Input: part model. Units: mm. Frame: model coordinates. Face numbers are marked on the shaded views. A direction names the side the tool comes from. Coordinates: 2 decimals unless noted, no trailing zeros. Order: outer loops, then holes, each group sorted by start corner. A loop starts at its lowest first (then second) coordinate and runs counter-clockwise, first axis right, second up. Notation, with made-up numbers: (19, 50) -> (64, 50) arc R22 ccw to (64, 77) -> close; hole circle Ø2 at (-28.5, 37.5). An arc over 180 degrees is marked (long way). Answer as CSV lines item,"result".
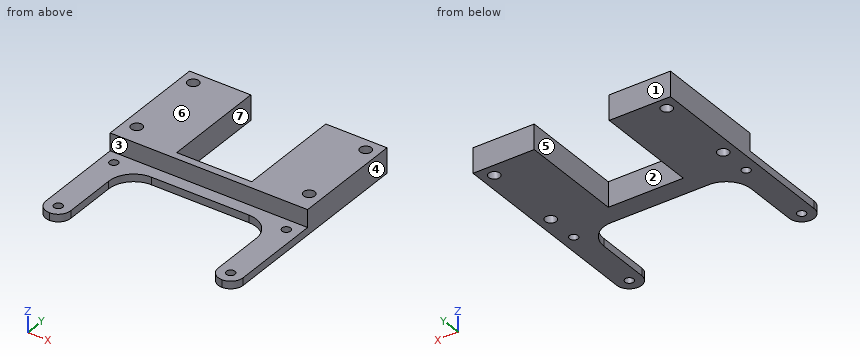
from build123d import *

# Parameters (mm, degrees)
BOSS_EXTRUDE1_DEPTH  = 3
FILLET1_R            = 10
FILLET2_R            = 5
M3_CLEARANCE_HOLE1_D = 3.4
BOSS_EXTRUDE3_DEPTH  = 10
M4_CLEARANCE_HOLE1_D = 4.5


with BuildPart() as part:
    # Sketch1 → Boss-Extrude1 (new body)
    with BuildSketch(Plane.XY):
        Polygon((28.024558014, 7.846809304), (28.024558014, -28.653190696), (38.024558014, -28.653190696), (38.024558014, 12.846809304), (-40.975441986, 12.846809304), (-40.975441986, -28.653190696), (-30.975441986, -28.653190696), (-30.975441986, 7.846809304), align=None)
    extrude(amount=BOSS_EXTRUDE1_DEPTH)

    # Fillet1
    fillet1_edges = [part.edges().sort_by_distance(p)[0] for p in [
        (28.024558014, 7.846809304, 1.5),
        (-30.975441986, 7.846809304, 1.5),
    ]]
    fillet(fillet1_edges, radius=FILLET1_R)

    # Fillet2
    fillet2_edges = [part.edges().sort_by_distance(p)[0] for p in [
        (-30.975441986, -28.653190696, 1.5),
        (-40.975441986, -28.653190696, 1.5),
        (28.024558014, -28.653190696, 1.5),
        (38.024558014, -28.653190696, 1.5),
    ]]
    fillet(fillet2_edges, radius=FILLET2_R - 0.0001)  # a hair under: the kernel refuses the full size

    # M3 Clearance Hole1 (through all)
    with Locations(Plane(origin=(0, 0, 0), x_dir=(-1, 0, 0), z_dir=(0, 0, -1))):
        with Locations((-33.024558014, 7.846809304), (35.975441986, -23.653190696), (35.975441986, 7.846809304), (-33.024558014, -23.653190696)):
            Hole(M3_CLEARANCE_HOLE1_D / 2)

    # Sketch5 → Boss-Extrude3 (add)
    with BuildSketch(Plane(origin=(0, 0, 0), x_dir=(-1, 0, 0), z_dir=(0, 0, -1))):
        Polygon((-38.024558014, 57.846809304), (-38.024558014, 12.846809304), (40.975441986, 12.846809304), (40.975441986, 57.846809304), (16.475441986, 57.846809304), (16.475441986, 15.846809304), (-13.524558014, 15.846809304), (-13.524558014, 57.846809304), align=None)
    extrude(amount=-BOSS_EXTRUDE3_DEPTH)

    # M4 Clearance Hole1 (through all)
    with Locations(Plane(origin=(0, 0, 0), x_dir=(-1, 0, 0), z_dir=(0, 0, -1))):
        with Locations((-33.024558014, 52.846809304), (-33.024558014, 20.846809304), (35.975441986, 20.846809304), (35.975441986, 52.846809304)):
            Hole(M4_CLEARANCE_HOLE1_D / 2)


solid = part.part
1. Reachability of the marked faces 1, 2 and 3 from +Z, -Z, +X, -X, +Y, -Y: full face, straight path, thin tool, end or side. Return the list, or none.
Findings:
face 1,"+Z, -Z, +X, -X, +Y"
face 2,"+Z, -Z, +Y"
face 3,"+Z, +X, -X, -Y"
2. Cut plane A-A (y = 41.5). Return the cut outline in (x, z), plus the area to 3 significant figures.
Findings:
outline,"(-40.98, 0) -> (-16.48, 0) -> (-16.48, 10) -> (-40.98, 10) -> close; (13.52, 0) -> (38.02, 0) -> (38.02, 10) -> (13.52, 10) -> close"
area,"490 mm2"
3. Cut plane D-D (z = 8). Return the cut outline in (x, y), plus the area to 3 significant figures.
Findings:
outline,"(-40.98, 12.85) -> (38.02, 12.85) -> (38.02, 57.85) -> (13.52, 57.85) -> (13.52, 15.85) -> (-16.48, 15.85) -> (-16.48, 57.85) -> (-40.98, 57.85) -> close; hole circle Ø4.5 at (-35.98, 20.85); hole circle Ø4.5 at (-35.98, 52.85); hole circle Ø4.5 at (33.02, 20.85); hole circle Ø4.5 at (33.02, 52.85)"
area,"2,230 mm2"
4. Ray query, line 1 along X through (y, z) = (33, 5); line 2 along X through (y, z) = (-3, 2.5); line 3 along Y through (x, z) = (-34, 2.75). Return the intervals inside material, ascending.
Findings:
line 1,"x = -40.98 to -16.48, 13.52 to 38.02"
line 2,"x = -40.98 to -30.98, 28.02 to 38.02"
line 3,"y = -28.25 to 19.77, 21.92 to 51.77, 53.92 to 57.85"
5. Cut plane B-B (z = 1.5). State how many separate pieces and enclosed holes the cut face has, plus the area to 3 significant figures.
Findings:
separate pieces,"1"
enclosed holes,"8"
area,"3,340 mm2"
6. Cut plane C-C (x = 2.5). Return the cut outline in (y, z), plus the area to 3 significant figures.
Findings:
outline,"(7.85, 0) -> (15.85, 0) -> (15.85, 10) -> (12.85, 10) -> (12.85, 3) -> (7.85, 3) -> close"
area,"45.0 mm2"
7. Mould query, pull axis X, two halves, no side actions, for the marked faces 4, 5, 6 and 7. Classes: released by +X, released by -X, zero draft, split by the parting line, or undercut.
Findings:
face 4,"released by +X"
face 5,"undercut"
face 6,"zero draft"
face 7,"undercut"
8. Contact query for flat-ended pins moving along their axis: pin 1 (2 mm diameter, centred on x = -35.98, y = 7.85, fed in from -Z); pin 2 (6 mm diameter, centred on x = 33.02, y = 20.85, fed in from -Z). Output: stop coordinate, or through.
Findings:
pin 1,"passes through"
pin 2,"stops at z = 0"
